from build123d import *

# Parameters (mm, degrees)
F1_DEPTH = 88.9
F3_DEPTH = 25.4
F4_ANGLE = -90


with BuildPart() as f1:
    # F0 (on Front) → F1 (new body)
    with BuildSketch(Plane.XZ):
        Polygon((21.59, 0), (0, 0), (0, -3.175), (21.59, -3.175), (28.3751536726, 3.6101536726), (37.3921536726, 3.6101536726), (37.3921536726, 1.256122898), (36.5982342043, -3.2464181487), (37.4145606636, -0.1998463274), (39.6781536726, -0.1998463274), (39.6781536726, 5.3881536726), (26.9781536726, 5.3881536726), align=None)
        with BuildLine():
            Line((36.5982342043, -3.2464181487), (37.3921536726, 1.256122898))
            ThreePointArc((37.3921536726, 1.256122898), (34.7439234151, -0.5981878912), (36.5982342043, -3.2464181487))
        make_face()
    extrude(amount=F1_DEPTH)

    # F2 (on face) → F3 (cut)
    with BuildSketch(Plane.XY):
        with BuildLine():
            Line((10.795, -22.225), (10.795, -15.875))
            Line((10.795, -15.875), (6.06425, -15.875))
            ThreePointArc((6.06425, -15.875), (2.88925, -19.05), (6.06425, -22.225))
            Line((6.06425, -22.225), (10.795, -22.225))
        make_face()
        with BuildLine():
            Line((15.52575, -15.875), (10.795, -15.875))
            Line((10.795, -15.875), (10.795, -22.225))
            Line((10.795, -22.225), (15.52575, -22.225))
            ThreePointArc((15.52575, -22.225), (18.70075, -19.05), (15.52575, -15.875))
        make_face()
        with BuildLine():
            Line((10.795, -73.025), (10.795, -66.675))
            Line((10.795, -66.675), (6.06425, -66.675))
            ThreePointArc((6.06425, -66.675), (2.88925, -69.85), (6.06425, -73.025))
            Line((6.06425, -73.025), (10.795, -73.025))
        make_face()
        with BuildLine():
            Line((15.52575, -66.675), (10.795, -66.675))
            Line((10.795, -66.675), (10.795, -73.025))
            Line((10.795, -73.025), (15.52575, -73.025))
            ThreePointArc((15.52575, -73.025), (18.70075, -69.85), (15.52575, -66.675))
        make_face()
    extrude(amount=-F3_DEPTH, mode=Mode.SUBTRACT)


with BuildPart() as f1_1:
    # F4: moved
    add(f1.part.rotate(Axis((10.795, 0, 0), (1, 0, 0)), F4_ANGLE))


solid = f1_1.part
Build history of the part. All positions in model axes, mm. A direction names the side the tool comes from. Round coordinates to 2 decimals unless told otherwise and drop trailing zeros. Loops run counter-clockwise (first coordinate to the right, second up) from the corner with the lowest first, then second, coordinate; pieces in that order, holes last. Notation, with made-up numbers: (-24.75, -5.75) -> (27.25, -5.75) arc R32 ccw to (27.25, 22.25) -> close; hole circle Ø11 at (-14, 22). An arc over 180 degrees is marked (long way). One line per item, written item: value. Start each with the question number.
Q1. 3-axis set-ups, long thin cutter, end or side, ignore diameter. For faces 1 (the face through (11, -2, 73.025)), 2 (the face through (11, -3.175, 44)), 3 (the face through (24.935, 0.17, 43.828)): which of +Z, -Z, +X, -X, +Y, -Y reach the whole face in a straight line?
Q2. Cut at A-A on z = 69.85. List the corners of the cut face in (x, y) (3 decimals), plus the area to 3 significant figures.
Q3. Cut at C-C on x = 24. List the corners of the cut face in (y, z) (3 decimals), plus the area to 3 significant figures.
Q4. Two-plate mould, pull along X, no slides. Class faces 4 (the face through (2.89, -1.57, 18.98)), 5 (the face through (33, 5.388, 44)), 6 (the face through (0, -2, 44)): released by +X, released by -X, zero draft, split by the parting line, or undercut.
Q5. Drop flat-ended pins along their axis: pin 1 Ø17.5 at (x, z) = (11.5, 39) entering from -Y (3 decimals); pin 2 Ø7 at (x, z) = (31, 28) entering from -Y (3 decimals); pin 3 Ø10 at (x, z) = (31, 10.5) entering from -Y. Give the stop position or say it passes through.
Q6. Cut at B-B on x = 13. List the corners of the cut face in (y, z) (3 decimals), plus the area to 3 significant figures.
Q7. Probe line 1 along Z through (x, y) = (9, -1) (3 decimals); line 2 along Z through (x, y) = (4, -1.5); line 3 along X through (y, z) = (-0.75, 19.5) (3 decimals). List the from-to ranges inside material, lowest first.
Computed:
1. face 1: +Y, -Y
1. face 2: +Z, -Z, -X, -Y
1. face 3: +Z, -Z, -Y
2. outline: (0, -3.175) -> (2.889, -3.175) -> (2.889, 0) -> (0, 0) -> close; (18.701, -3.175) -> (21.59, -3.175) -> (28.375, 3.61) -> (37.392, 3.61) -> (37.392, 1.256) arc R2.286 ccw to (36.598, -3.246) -> (37.415, -0.2) -> (39.678, -0.2) -> (39.678, 5.388) -> (26.978, 5.388) -> (21.59, 0) -> (18.701, 0) -> close
2. area: 76.5 mm²
3. outline: (-0.765, 0) -> (2.41, 0) -> (2.41, 88.9) -> (-0.765, 88.9) -> close
3. area: 282 mm²
4. face 4: undercut
4. face 5: zero draft
4. face 6: released by -X
5. pin 1: y = -3.175
5. pin 2: y = 2.735
5. pin 3: y = -3.05
6. outline: (-3.175, 0) -> (0, 0) -> (0, 15.875) -> (-3.175, 15.875) -> close; (-3.175, 22.225) -> (0, 22.225) -> (0, 66.675) -> (-3.175, 66.675) -> close; (-3.175, 73.025) -> (0, 73.025) -> (0, 88.9) -> (-3.175, 88.9) -> close
6. area: 242 mm²
7. line 1: 0 to 15.875, 22.225 to 66.675, 73.025 to 88.9
7. line 2: 0 to 16.64, 21.46 to 67.44, 72.26 to 88.9
7. line 3: 0 to 2.921, 18.669 to 24.015, 34.722 to 37.267
